Geometry check sheet. Reference: the model listing, model coordinates, mm. Face numbers are marked on the shaded views. A direction names the side the tool comes from. Give positions to 0.01 mm unless a question says otherwise; leave off trailing zeros. Write each loop counter-clockwise with the first axis right and the second up, starting at its lowest first coordinate (ties: lowest second). Pieces come first, ordered by that corner, then holes. Notation, with made-up numbers: (24, -17.5) - (60, -17.5) arc R18 cw to (60, 9.5) - close; hole circle Ø5 at (-2, 16). An arc over 180 degrees is marked (long way). Write item = value, one per line. Start each with the question number.
(1) Section check C-C, the plane y = -5.5. Enter the section's corners in (x, z).
(2) Section check D-D, the plane x = -4.25. Enter the section's corners in (y, z).
(3) Depth check by flat-ended pin: pin 1 Ø3 at (y, z) = (-3.5, -8) entering from -X; pin 2 Ø5 at (x, y) = (-7.5, -6) entering from -Z; pin 3 Ø12 at (x, z) = (-11, 10) entering from +Y; pin 4 Ø2.5 at (x, z) = (0, 0) entering from +Y. Enter the tip coordinate at first touch or a pass-through.
(4) Thickness scan on L1, parallel to X at y = -1.5, z = -6; L2, parallel to Z at x = -10.25, y = -5; L3, parallel to Y at x = -6, z = 8. Record the ranges inside material, lowest first.
(5) Section check B-B, the plane z = 0. Enter the section's corners in (x, y), plus the area to 3 significant figures.
(6) Section check A-A, the plane x = 0. Enter the section's corners in (y, z), plus the area to 3 significant figures.
(7) Access from +Z, -Z, +X, -X, +Y, -Y to the whole of each face (thin tool, end or side, straight path). Record for the marked faces 1, 2 and 3.
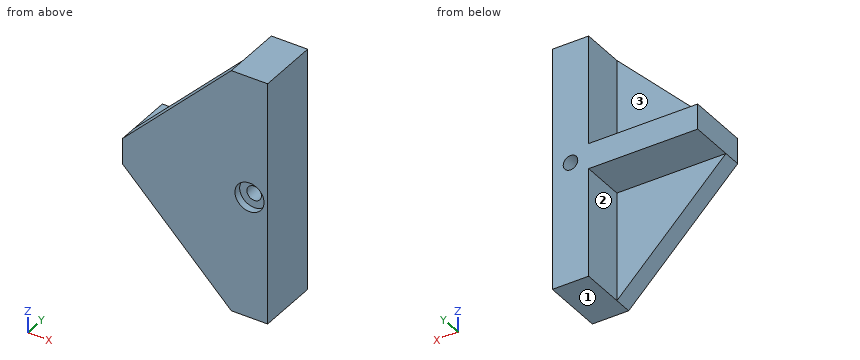
```python
from build123d import *

# Parameters (mm, degrees)
F1_DEPTH = 6
F3_DEPTH = 2.5
F4_R     = 1
F5_DEPTH = 8.501
F6_R     = 2
F7_DEPTH = 1


with BuildPart() as f1:
    # F0 (on Front) → F1 (new body)
    with BuildSketch(Plane.XZ):
        Polygon((2.5, 1), (2.5, 16.75), (-2.5, 16.75), (-2.5, 1.75), (-17.5, 1.75), (-17.5, -1.75), (-2.5, -1.75), (-2.5, -16.75), (2.5, -16.75), (2.5, -2.5), align=None)
    extrude(amount=F1_DEPTH)

    # F2 (on face) → F3 (join)
    with BuildSketch(Plane.XZ.offset(6)):
        Polygon((-2.5, 16.75), (-17.5, 1.75), (-17.5, 0), (-17.5, -1.75), (-2.5, -16.75), (0, -16.75), (2.5, -16.75), (2.5, 16.75), (0, 16.75), align=None)
    extrude(amount=F3_DEPTH)

    # F4 (on face) → F5 (cut, through all)
    with BuildSketch(Plane(origin=(0, 0, 0), x_dir=(-1, 0, 0), z_dir=(0, 1, 0))):
        Circle(F4_R)
    extrude(amount=-F5_DEPTH, mode=Mode.SUBTRACT)

    # F6 (on face) → F7 (cut)
    with BuildSketch(Plane.XZ.offset(8.5)):
        Circle(F6_R)
    extrude(amount=-F7_DEPTH, mode=Mode.SUBTRACT)


solid = f1.part
```
Model answer:
q1.outline = (-17.5, -1.75) - (-2.5, -1.75) - (-2.5, -16.75) - (2.5, -16.75) - (2.5, 16.75) - (-2.5, 16.75) - (-2.5, 1.75) - (-17.5, 1.75) - close; hole circle Ø2 at (0, 0)
q2.outline = (-8.5, -15) - (-6, -15) - (-6, -1.75) - (0, -1.75) - (0, 1.75) - (-6, 1.75) - (-6, 15) - (-8.5, 15) - close
q3.pin_1 = -2.5
q3.pin_2 = -14.25
q3.pin_3 = -6
q3.pin_4 = 0
q4.L1 = -2.5 to 2.5
q4.L2 = -1.75 to 1.75
q4.L3 = -8.5 to -6
q5.outline = (-17.5, -8.5) - (-2, -8.5) - (-2, -7.5) - (-1, -7.5) - (-1, 0) - (-17.5, 0) - close; (1, -7.5) - (2, -7.5) - (2, -8.5) - (2.5, -8.5) - (2.5, 0) - (1, 0) - close
q5.area = 151 mm²
q6.outline = (-8.5, -16.75) - (0, -16.75) - (0, -1) - (-7.5, -1) - (-7.5, -2) - (-8.5, -2) - close; (-8.5, 2) - (-7.5, 2) - (-7.5, 1) - (0, 1) - (0, 16.75) - (-8.5, 16.75) - close
q6.area = 266 mm²
q7.face_1 = -Z, +X, -X, +Y, -Y
q7.face_2 = -Z, -X, +Y
q7.face_3 = +Z, -X, +Y
